Geometry check sheet. Reference: the model listing, model coordinates, mm. Face numbers are marked on the shaded views. A direction names the side the tool comes from. Round coordinates to 2 decimals unless told otherwise and drop trailing zeros. Loops run counter-clockwise (first coordinate to the right, second up) from the corner with the lowest first, then second, coordinate; pieces in that order, holes last.
```python
from build123d import *

# Parameters (mm, degrees)
BOSS_EXTRUDE1_DEPTH = 2
BOSS_EXTRUDE2_DEPTH = 13
BOSS_EXTRUDE3_DEPTH = 5
SKETCH8_R           = 1.5
CUT_EXTRUDE3_DEPTH  = 30.954131602
SKETCH10_W          = 12.2
SKETCH10_H          = 12.2
BOSS_EXTRUDE4_DEPTH = 0.8
SKETCH11_R          = 0.925
CUT_EXTRUDE4_DEPTH  = 38.013511047
SKETCH12_R          = 1.05
CUT_EXTRUDE5_DEPTH  = 38.01351122


with BuildPart() as part:
    # Sketch1 → Boss-Extrude1 (new body)
    with BuildSketch(Plane(origin=(0, 0, 0), x_dir=(1, 0, 0), z_dir=(0, 1, 0))):
        with BuildLine():
            Line((-9.5, 11.5), (9.5, 11.5))
            ThreePointArc((9.5, 11.5), (21, 0), (9.5, -11.5))
            Line((9.5, -11.5), (-9.5, -11.5))
            ThreePointArc((-9.5, -11.5), (-21, 0), (-9.5, 11.5))
        make_face()
    extrude(amount=BOSS_EXTRUDE1_DEPTH)

    # Sketch2 → Boss-Extrude2 (add)
    with BuildSketch(Plane(origin=(0, 2, 0), x_dir=(1, 0, 0), z_dir=(0, 1, 0))):
        with BuildLine():
            ThreePointArc((-9.5, 11.5), (-21, 0), (-9.5, -11.5))
            Line((-9.5, -11.5), (9.5, -11.5))
            ThreePointArc((9.5, -11.5), (21, 0), (9.5, 11.5))
            Line((9.5, 11.5), (-9.5, 11.5))
        make_face()
        with BuildLine():
            ThreePointArc((-9.5, 9.5), (-4.876689498, 8.299096336), (-1.422252789, 5))
            Line((-1.422252789, 5), (1.422252789, 5))
            ThreePointArc((1.422252789, 5), (4.876689498, 8.299096336), (9.5, 9.5))
            ThreePointArc((9.5, 9.5), (19, 0), (9.5, -9.5))
            ThreePointArc((9.5, -9.5), (4.876689498, -8.299096336), (1.422252789, -5))
            Line((1.422252789, -5), (-1.422252789, -5))
            ThreePointArc((-1.422252789, -5), (-4.876689498, -8.299096336), (-9.5, -9.5))
            ThreePointArc((-9.5, -9.5), (-19, 0), (-9.5, 9.5))
        make_face(mode=Mode.SUBTRACT)
    extrude(amount=BOSS_EXTRUDE2_DEPTH)

    # Sketch4 → Boss-Extrude3 (add)
    with BuildSketch(Plane(origin=(0, 15, 0), x_dir=(1, 0, 0), z_dir=(0, 1, 0))):
        with BuildLine():
            Line((9.5, 11.5), (-9.5, 11.5))
            ThreePointArc((-9.5, 11.5), (-21, 0), (-9.5, -11.5))
            Line((-9.5, -11.5), (9.5, -11.5))
            ThreePointArc((9.5, -11.5), (21, 0), (9.5, 11.5))
        make_face()
        with BuildLine():
            Line((9.5, 10.5), (-9.5, 10.5))
            ThreePointArc((-9.5, 10.5), (-20, 0), (-9.5, -10.5))
            Line((-9.5, -10.5), (9.5, -10.5))
            ThreePointArc((9.5, -10.5), (20, 0), (9.5, 10.5))
        make_face(mode=Mode.SUBTRACT)
    extrude(amount=BOSS_EXTRUDE3_DEPTH)

    # Sketch8 → Cut-Extrude3 (cut, through all)
    with BuildSketch(Plane(origin=(0, 2, 0), x_dir=(1, 0, 0), z_dir=(0, 1, 0))):
        with Locations(Location((-9.5, 0, 0), (0, 0, 270))):
            Circle(SKETCH8_R)
        with Locations(Location((9.5, 0, 0), (0, 0, 90))):
            Circle(SKETCH8_R)
    extrude(amount=-CUT_EXTRUDE3_DEPTH, mode=Mode.SUBTRACT)

    # Sketch10 → Boss-Extrude4 (add)
    with BuildSketch(Plane(origin=(0, 2, 0), x_dir=(1, 0, 0), z_dir=(0, 1, 0))):
        with BuildLine():
            Line((-1.422252789, -5), (1.422252789, -5))
            ThreePointArc((1.422252789, -5), (19, 0), (1.422252789, 5))
            Line((1.422252789, 5), (-1.422252789, 5))
            ThreePointArc((-1.422252789, 5), (-19, 0), (-1.422252789, -5))
        make_face()
        with Locations((9.5, 0)):
            Rectangle(SKETCH10_W, SKETCH10_H, mode=Mode.SUBTRACT)
        with Locations((-9.5, 0)):
            Rectangle(SKETCH10_W, SKETCH10_H, mode=Mode.SUBTRACT)
    extrude(amount=BOSS_EXTRUDE4_DEPTH)

    # Sketch11 → Cut-Extrude4 (cut, through all)
    with BuildSketch(Plane.XY.offset(11.5)):
        with Locations((-5.4, 3.9)):
            Circle(SKETCH11_R)
        with Locations((-13.6, 3.9)):
            Circle(SKETCH11_R)
        with Locations((13.6, 3.9)):
            Circle(SKETCH11_R)
        with Locations((5.4, 3.9)):
            Circle(SKETCH11_R)
    extrude(amount=-CUT_EXTRUDE4_DEPTH, mode=Mode.SUBTRACT)

    # Sketch12 → Cut-Extrude5 (cut, through all)
    with BuildSketch(Plane.XY.offset(11.5)):
        with Locations((0, 17.5)):
            Circle(SKETCH12_R)
    extrude(amount=-CUT_EXTRUDE5_DEPTH, mode=Mode.SUBTRACT)


solid = part.part
```
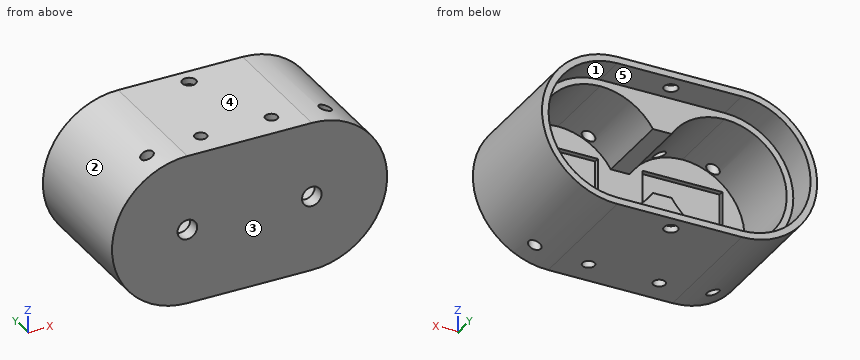
1) Access from +Z, -Z, +X, -X, +Y, -Y to the whole of each face (thin tool, end or side, straight path). Record for the marked faces 4 and 5.
Report:
face 4: +Z, +X, -X, +Y, -Y
face 5: +Y
2) Sectioned sample at C-C, the plane x = -8.5. Record the cut outline in (y, z).
Report:
outline: (0, -11.5) - (20, -11.5) - (20, -10.5) - (15, -10.5) - (15, -9.45) - (2.8, -9.45) - (2.8, -6.1) - (2, -6.1) - (2, -1.12) - (0, -1.12) - close; (0, 1.12) - (2, 1.12) - (2, 6.1) - (2.8, 6.1) - (2.8, 9.45) - (15, 9.45) - (15, 10.5) - (20, 10.5) - (20, 11.5) - (0, 11.5) - close
3) Sectioned sample at B-B, the plane y = 9. Record the cut outline in (x, z).
Report:
outline: (-9.5, -11.5) - (9.5, -11.5) arc R11.5 ccw to (9.5, 11.5) - (-9.5, 11.5) arc R11.5 ccw to start; hole (-1.42, -5) - (1.42, -5) arc R9.5 ccw (long way) to (1.42, 5) - (-1.42, 5) arc R9.5 ccw (long way) to start
4) Sectioned sample at A-A, the plane x = 0. Record the cut outline in (y, z), then the cut area to 3 significant figures.
Report:
outline: (0, -11.5) - (16.45, -11.5) - (16.45, -10.5) - (15, -10.5) - (15, -5) - (2.8, -5) - (2.8, 5) - (15, 5) - (15, 10.5) - (16.45, 10.5) - (16.45, 11.5) - (0, 11.5) - close; (18.55, -11.5) - (20, -11.5) - (20, -10.5) - (18.55, -10.5) - close; (18.55, 10.5) - (20, 10.5) - (20, 11.5) - (18.55, 11.5) - close
area: 229 mm2
5) Sectioned sample at D-D, the plane z = -0.25. Record the cut outline in (x, y).
Report:
outline: (-21, 0) - (-10.98, 0) - (-10.98, 2) - (-15.6, 2) - (-15.6, 2.8) - (-19, 2.8) - (-19, 15) - (-20, 15) - (-20, 20) - (-21, 20) - close; (-8.02, 0) - (8.02, 0) - (8.02, 2) - (3.4, 2) - (3.4, 2.8) - (-3.4, 2.8) - (-3.4, 2) - (-8.02, 2) - close; (10.98, 0) - (21, 0) - (21, 20) - (20, 20) - (20, 15) - (19, 15) - (19, 2.8) - (15.6, 2.8) - (15.6, 2) - (10.98, 2) - close
6) Scan lines: line 1 along X through (y, z) = (4, -9.75); line 2 along Y through (x, z) = (13.6, -10.3) (3 decimals); line 3 along Y through (x, z) = (-5.4, -9.35) (3 decimals). Record each from-to range of solid material in increasing order.
Report:
line 1: x = -15.6 to -14.52, -12.68 to -6.32, -4.48 to 4.48, 6.32 to 12.68, 14.52 to 15.6
line 2: y = 0 to 2.975, 4.825 to 20
line 3: y = 0 to 2.975, 4.825 to 15
7) Mould release check, pull along Z, two halves, no side actions. Record for the marked faces 1, 2 and 3: +Z half, -Z half, draft (parallel to the pull), parting line (faces both ways), or undercut.
Report:
face 1: undercut
face 2: parting line
face 3: draft
8) Gauge pin test, flat ends, axial feed: pin 1 (0.9 mm diameter, centred on y = 2.5, z = 1.5, fed in from +X); pin 2 (2 mm diameter, centred on x = 13.6, y = 3.9, fed in from +Z); pin 3 (6 mm diameter, centred on x = -10, z = 1, fed in from +Y). Record the tip position at first contact, or that the pin passes through.
Report:
pin 1: stops at x = 20.95
pin 2: stops at z = 11.07
pin 3: stops at y = 2
